```python
from build123d import *

# Parameters (mm, degrees)
F1_DEPTH = 3


# Not quite as in the source:
# - ends of sketch curves that miss each other by under 0.0002 mm in the source are joined


with BuildPart() as f1:
    # F0 (on Right) → F1 (new body)
    with BuildSketch(Plane.YZ):
        Polygon((-16.4821194199, 3.4866289613), (-19.4821194199, 3.4866289613), (-19.4821194199, -0.0133710387), (-19.4821194199, -3.5133710387), (-16.4821194199, -3.5133710387), (-16.4821194218, -13.5133710387), (-19.4821194199, -13.5133710387), (-19.4821194222, -20.5133710387), (-12.4821194199, -20.5133710387), (-12.4821194214, -23.5133710387), (-2.4821194199, -23.5133710387), (-2.4821194202, -20.5133710387), (-0.9821194199, -20.5133710387), (-0.98211942, -14.0133710387), (-1.9821194199, -14.0133710387), (-1.9821194199, -12.0667160037), (-0.9821194199, -12.0667160037), (-0.98211942, -8.5667160037), (-0.0066117616, -8.5667160037), (0.0178805801, -8.5667160037), (0.9933873842, -8.5654249595), (0.9979620612, -12.0654219699), (1.997962061, -12.0654219699), (2.0005064375, -14.0120753421), (1.0005064375, -14.0120753421), (1.0090022661, -20.5120697898), (2.5090009847, -20.510109214), (2.5129221366, -23.5101066514), (12.5129135944, -23.4970361461), (12.5089924443, -20.4970387087), (19.5089864635, -20.4878893549), (19.499837112, -13.4878953343), (16.4998396723, -13.4918164859), (16.4867691689, -3.4918250278), (19.4867666044, -3.4879038762), (19.4821919275, 0.0120931341), (19.4776172507, 3.5120901445), (16.4776198132, 3.5081689929), (16.4645493098, 13.508160451), (19.4645467453, 13.5120816026), (19.4553973939, 20.5120756232), (12.4554033709, 20.5029262695), (12.4514822208, 23.5029237069), (2.4514907612, 23.4898532016), (2.4554119131, 20.4898557642), (0.9554131941, 20.4878951884), (0.9639090227, 13.9879007406), (1.9639081685, 13.9892077911), (1.9639081683, 12.0425510933), (0.9664533991, 12.0412473684), (0.9710280761, 8.5412503581), (0.0178805401, 8.540004545), (-0.0289710698, 8.5399739263), (-0.9821194199, 8.5399739263), (-0.9821194199, 12.0399739263), (-1.9821194199, 12.0399739263), (-1.9821194199, 13.9866289613), (-0.9821194199, 13.9866289613), (-0.9821194199, 20.4866289613), (-2.4821194199, 20.4866289613), (-2.4821194199, 23.4866289613), (-12.4821194199, 23.4866289613), (-12.4821194199, 20.4866289613), (-19.4821194199, 20.4866289613), (-19.4821194199, 13.4866289613), (-16.4821194199, 13.4866289613), align=None)
    extrude(amount=F1_DEPTH)


solid = f1.part
```
Build history of the part. All positions in model axes, mm. A direction names the side the tool comes from. Round coordinates to 2 decimals unless told otherwise and drop trailing zeros. Loops run counter-clockwise (first coordinate to the right, second up) from the corner with the lowest first, then second, coordinate; pieces in that order, holes last.
Item 1: Saw through at A-A (z = 15.5). List the corners of the cut face in (x, y).
Item 2: Drill centre lines: line 1 along Z through (x, y) = (0.5, -17); line 2 along Y through (x, z) = (2, 16.5); line 3 along Y through (x, z) = (2.5, 9). Where is each one in solid material? Low to high.
Item 3: Saw through at B-B (y = -15). List the corners of the cut face in (x, z), then the cut area to 3 significant figures.
Item 4: Which spindle directions (+Z, -Z, +X, -X, +Y, -Y) get a long thin tool onto all of the face, cutting with end or side? Do faces 4 (the face through (1.5, -1.5, 12.04)), 5 (the face through (1, -18, -3.513)), 6 (the face through (1, -0.982, -17)). Say none if no direction does.
Item 5: Pin check, flat tips, straight feed: P1, Ø1.5, axis at x = 1.5, z = -8, coming from the -Y side; P2, Ø0.5, axis at x = 1.5, y = -0.5, coming from the +Z side; P3, Ø1.5, axis at x = 1, z = 17.5, coming from the +Y side; P4, Ø3, axis at y = 0, z = 17, coming from the +X side. Stop position of each tip, or through.
Item 6: Saw through at C-C (z = 5). List the corners of the cut face in (x, y), then the cut area to 3 significant figures.
Item 7: Two-plate mould, pull along Z, no slides. Class faces 1 (the face through (1, -16, -20.513)), 2 (the face through (1, 1.964, 13)), 3 (the face through (3, 0, 0)): released by +Z, released by -Z, zero draft, split by the parting line, or undercut.
Worked answers:
1. outline: (0, -19.48) - (3, -19.48) - (3, -0.98) - (0, -0.98) - close; (0, 0.96) - (3, 0.96) - (3, 19.46) - (0, 19.46) - close
2. line 1: z = -20.51 to -13.51, -3.51 to 3.49, 13.49 to 20.49
2. line 2: y = -19.48 to -0.98, 0.96 to 19.46
2. line 3: y = -16.48 to -0.98, 0.97 to 16.47
3. outline: (0, -20.51) - (3, -20.51) - (3, 20.49) - (0, 20.49) - close
3. area: 123 mm2
4. face 4: +X, -X
4. face 5: +X, -X, -Y
4. face 6: -Z, +X, -X
5. P1: stops at y = -16.48
5. P2: stops at z = 8.54
5. P3: stops at y = 19.46
5. P4: stops at x = 3
6. outline: (0, -16.48) - (3, -16.48) - (3, 16.48) - (0, 16.48) - close
6. area: 98.9 mm2
7. face 1: released by -Z
7. face 2: undercut
7. face 3: zero draft
